from build123d import *

# Parameters (mm, degrees)
SKETCH2_W                = 200
SKETCH2_H                = 200
BOSS_EXTRUDE1_DEPTH      = 10
SKETCH12_R               = 90
SKETCH12_R_2             = 85
CUT_EXTRUDE8_DEPTH       = 4
SKETCH13_R               = 1
CUT_EXTRUDE9_DEPTH       = 142.774468788
SKETCH4_W                = 200
SKETCH4_H                = 200
SKETCH4_W_2              = 174
SKETCH4_H_2              = 174
BOSS_EXTRUDE4_DEPTH      = 60
CUT_EXTRUDE10_DEPTH      = 232.516738056
CUT_EXTRUDE10_DEPTH_BACK = 232.516738056
CUT_EXTRUDE11_DEPTH      = 232.516738056
CUT_EXTRUDE11_DEPTH_BACK = 232.516738056
CUT_EXTRUDE12_DEPTH      = 10
SKETCH19_W               = 200
SKETCH19_H               = 200
BOSS_EXTRUDE5_DEPTH      = 10


with BuildPart() as part:
    # Sketch2 → Boss-Extrude1 (new body)
    with BuildSketch(Plane(origin=(0, 0, 0), x_dir=(1, 0, 0), z_dir=(0, 1, 0))):
        Rectangle(SKETCH2_W, SKETCH2_H)
    extrude(amount=BOSS_EXTRUDE1_DEPTH)

    # Sketch12 → Cut-Extrude8 (cut)
    with BuildSketch(Plane(origin=(0, 10, 0), x_dir=(1, 0, 0), z_dir=(0, 1, 0))):
        with Locations(Location((0, 0, 0), (0, 0, 270))):
            Circle(SKETCH12_R)
        with Locations(Location((0, 0, 0), (0, 0, 270))):
            Circle(SKETCH12_R_2, mode=Mode.SUBTRACT)
    extrude(amount=-CUT_EXTRUDE8_DEPTH, mode=Mode.SUBTRACT)

    # Sketch13 → Cut-Extrude9 (cut, through all)
    with BuildSketch(Plane(origin=(0, 10, 0), x_dir=(1, 0, 0), z_dir=(0, 1, 0))):
        with Locations(Location((0, 17, 0), (0, 0, 270))):
            Circle(SKETCH13_R)
        with Locations(Location((17, 0, 0), (0, 0, 270))):
            Circle(SKETCH13_R)
        with Locations(Location((0, -17, 0), (0, 0, 270))):
            Circle(SKETCH13_R)
        with Locations(Location((-17, 0, 0), (0, 0, 270))):
            Circle(SKETCH13_R)
    extrude(amount=-CUT_EXTRUDE9_DEPTH, mode=Mode.SUBTRACT)

    # Sketch4 → Boss-Extrude4 (add)
    with BuildSketch(Plane.XZ):
        Rectangle(SKETCH4_W, SKETCH4_H)
        Rectangle(SKETCH4_W_2, SKETCH4_H_2, mode=Mode.SUBTRACT)
    extrude(amount=BOSS_EXTRUDE4_DEPTH)

    # Sketch14 → Cut-Extrude10 (cut, two sides: drawn at the far end of the back side and taken through both)
    with BuildSketch(Plane.XY.offset(100).offset(-CUT_EXTRUDE10_DEPTH_BACK)):
        Polygon((0, -15), (70, -15), (70, -60), (-70, -60), (-70, -15), align=None)
    extrude(amount=CUT_EXTRUDE10_DEPTH + CUT_EXTRUDE10_DEPTH_BACK, mode=Mode.SUBTRACT)

    # Sketch15 → Cut-Extrude11 (cut, two sides: drawn at the far end of the back side and taken through both)
    with BuildSketch(Plane.ZY.offset(100).offset(-CUT_EXTRUDE11_DEPTH_BACK)):
        Polygon((0, -60), (-70, -60), (-70, -15), (70, -15), (70, -60), align=None)
    extrude(amount=CUT_EXTRUDE11_DEPTH + CUT_EXTRUDE11_DEPTH_BACK, mode=Mode.SUBTRACT)

    # Sketch3 → Cut-Extrude12 (cut)
    with BuildSketch(Plane(origin=(0, 10, 0), x_dir=(1, 0, 0), z_dir=(0, 1, 0))):
        with BuildLine():
            ThreePointArc((-38.01797101, -12.435187183), (0, -40), (38.01797101, -12.435187183))
            ThreePointArc((38.01797101, -12.435187183), (47.477938171, -7.638415216), (52.274710139, -17.098382377))
            ThreePointArc((52.274710139, -17.098382377), (0, -55), (-52.274710139, -17.098382377))
            ThreePointArc((-52.274710139, -17.098382377), (-47.477938171, -7.638415216), (-38.01797101, -12.435187183))
        make_face()
        with BuildLine():
            ThreePointArc((38.01797101, 12.435187183), (47.477938171, 7.638415216), (52.274710139, 17.098382377))
            ThreePointArc((52.274710139, 17.098382377), (0, 55), (-52.274710139, 17.098382377))
            ThreePointArc((-52.274710139, 17.098382377), (-47.477938171, 7.638415216), (-38.01797101, 12.435187183))
            ThreePointArc((-38.01797101, 12.435187183), (0, 40), (38.01797101, 12.435187183))
        make_face()
    extrude(amount=-CUT_EXTRUDE12_DEPTH, mode=Mode.SUBTRACT)

    # Sketch19 → Boss-Extrude5 (add)
    with BuildSketch(Plane.XZ.offset(60)):
        Rectangle(SKETCH19_W, SKETCH19_H)
    extrude(amount=BOSS_EXTRUDE5_DEPTH)


solid = part.part
Design review of the part built by this model. Coordinates are the model's own, in mm. A direction names the side the tool comes from. Round coordinates to 2 decimals unless told otherwise and drop trailing zeros. Write each loop counter-clockwise with the first axis right and the second up, starting at its lowest first coordinate (ties: lowest second). Pieces come first, ordered by that corner, then holes.
Item 1: Consider section D-D on y = -11.5. Give the boundary of the cut face in (x, z), and give its area (3 significant figures).
Item 2: Wall thickness on L1, parallel to X at y = 9, z = 0; L2, parallel to X at y = 5.5, z = 0; L3, parallel to Y at x = -51.5, z = -42.5: over which ranges is each line inside the solid? List them lowest first.
Item 3: For faces 5 (the flat face through (-70, -38, -94)), 6 (the flat face through (-1, 0, -1)), 7 (the flat face through (94, -15, -1)), 8 (the flat face through (-1, 10, -1)), 9 (the cylindrical face through (0.97, 5.07, -54.99)), list the 3-axis set-ups (+Z, -Z, +X, -X, +Y, -Y) from which the entire face can be reached by the end or side of a thin tool; tool diameter is ignored.
Item 4: Consider section C-C on x = 60. Give the boundary of the cut face in (y, z).
Item 5: For pin 1 Ø1.8 at (x, z) = (17, 0) entering from +Y, flat-tipped, find the tip position at first contact; note if it passes through.
Item 6: Consider section B-B on z = -77.5. Give the boundary of the cut face in (x, y), and give its area (3 significant figures).
Item 7: Consider section A-A on y = -30. Give the boundary of the cut face in (x, z), and give its area (3 significant figures).
Item 8: Draft analysis for pull direction Z (two halves, no side actions). For faces 1 (the cylindrical face through (47.32, 5.07, 7.59)), 2 (the flat face through (-1, -12, -100)), 3 (the cylindrical face through (0.97, 5.07, 54.99)), 4 (the flat face through (100, -12, -1)), state which applies: released by +Z, released by -Z, zero draft, split by the parting line, or undercut.
Check values:
1. outline: (-100, -100) - (100, -100) - (100, 100) - (-100, 100) - close; hole (-87, -87) - (87, -87) - (87, 87) - (-87, 87) - close
1. area: 9,720 mm2
2. L1: x = -100 to -90, -85 to -18, -16 to 16, 18 to 85, 90 to 100
2. L2: x = -100 to -18, -16 to 16, 18 to 100
2. L3: y = -70 to -60, 0 to 10
3. face 5: +Z, -Z
3. face 6: none
3. face 7: +X, -X
3. face 8: +Z, -Z, +X, -X, +Y
3. face 9: +Y
4. outline: (-70, -100) - (-60, -100) - (-60, 100) - (-70, 100) - close; (-15, -100) - (10, -100) - (10, -67.08) - (6, -67.08) - (6, -60.21) - (10, -60.21) - (10, 60.21) - (6, 60.21) - (6, 67.08) - (10, 67.08) - (10, 100) - (-15, 100) - (-15, 87) - (0, 87) - (0, -87) - (-15, -87) - close
5. pin 1: stops at y = -60
6. outline: (-100, -70) - (100, -70) - (100, 10) - (45.76, 10) - (45.76, 6) - (34.91, 6) - (34.91, 10) - (-34.91, 10) - (-34.91, 6) - (-45.76, 6) - (-45.76, 10) - (-100, 10) - close; hole (-87, -60) - (87, -60) - (87, 0) - (-87, 0) - close
6. area: 5,470 mm2
7. outline: (-100, -100) - (-70, -100) - (-70, -87) - (-87, -87) - (-87, -70) - (-100, -70) - close; (-100, 70) - (-87, 70) - (-87, 87) - (-70, 87) - (-70, 100) - (-100, 100) - close; (70, -100) - (100, -100) - (100, -70) - (87, -70) - (87, -87) - (70, -87) - close; (70, 87) - (87, 87) - (87, 70) - (100, 70) - (100, 100) - (70, 100) - close
7. area: 2,440 mm2
8. face 1: undercut
8. face 2: released by -Z
8. face 3: undercut
8. face 4: zero draft
